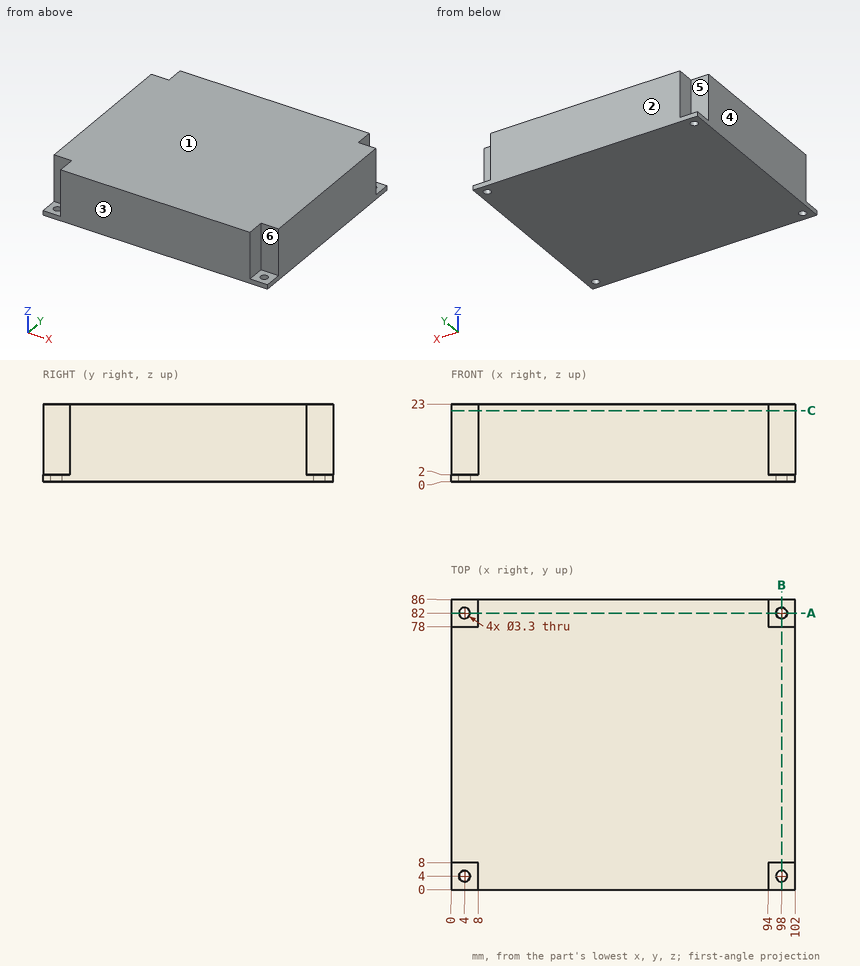
Design review of the part shown in the three views and the two pictorial views. Dimensions are in mm from the part's minimum x, y and z. A direction names the side the tool comes from. Give positions to 0.01 mm unless a question says otherwise; leave off trailing zeros. Write each loop counter-clockwise with the first axis right and the second up, starting at its lowest first coordinate (ties: lowest second). Pieces come first, ordered by that corner, then holes. Notation, with made-up numbers: M 17.5,43 L 25.5,43 A13 cw 25.5,64 Z; hole C -11.5,53 d6. An arc over 180 degrees is marked long. Return JSON: item names as keys, results as strings. Group by question number.
Item 1: Wall thickness on line 1 along Y through (x, z) = (4, 1.2); line 2 along X through (y, z) = (4, 0.85); line 3 along X through (y, z) = (81.5, 6.75): over which ranges is each line inside the solid? List them lowest first.
Item 2: Take a section at B-B (x = 98). Give the boundary of the cut face in (y, z), plus the area to 3 significant figures.
Item 3: Clearance check with flat-ended pins moving along their axes: pin 1 Ø2.5 at (x, y) = (3, 3) entering from +Z; pin 2 Ø6.5 at (x, z) = (98.5, 7.5) entering from -Y; pin 3 Ø4 at (x, z) = (5, 12.5) entering from +Y. State where each tip first meets the part, or that it passes through.
Item 4: The part is to be moulded in two halves that separate along Y. For the marked faces 1, 2 and 3, say which applies: pulls with the +Y half, pulls with the -Y half, needs draft (parallel to the pull), parting line crosses it, or undercut.
Item 5: Tool access review of the marked faces 4, 5 and 6: name each direction out of +Z, -Z, +X, -X, +Y, -Y from which nothing blocks a thin tool from reaching the whole face with its end or side.
Item 6: Take a section at A-A (y = 82). Give the boundary of the cut face in (x, z).
Item 7: Take a section at C-C (z = 21). Give the boundary of the cut face in (x, y).
Return value:
{
 "1": {"line 1": "y = 0 to 2.35, 5.65 to 80.35, 83.65 to 86", "line 2": "x = 0 to 2.35, 5.65 to 96.35, 99.65 to 102", "line 3": "x = 8 to 94"},
 "2": {"outline": "M 0,0 L 2.35,0 L 2.35,2 L 0,2 Z; M 5.65,0 L 80.35,0 L 80.35,2 L 78,2 L 78,23 L 8,23 L 8,2 L 5.65,2 Z; M 83.65,0 L 86,0 L 86,2 L 83.65,2 Z", "area": "1,630 mm2"},
 "3": {"pin 1": "stops at z = 2", "pin 2": "stops at y = 8", "pin 3": "stops at y = 78"},
 "4": {"face 1": "needs draft", "face 2": "pulls with the +Y half", "face 3": "pulls with the -Y half"},
 "5": {"face 4": "+Z, -Z, -X, +Y, -Y", "face 5": "+Z, -X, +Y", "face 6": "+Z, +X, -Y"},
 "6": {"outline": "M 0,0 L 2.35,0 L 2.35,2 L 0,2 Z; M 5.65,0 L 96.35,0 L 96.35,2 L 94,2 L 94,23 L 8,23 L 8,2 L 5.65,2 Z; M 99.65,0 L 102,0 L 102,2 L 99.65,2 Z"},
 "7": {"outline": "M 0,8 L 8,8 L 8,0 L 94,0 L 94,8 L 102,8 L 102,78 L 94,78 L 94,86 L 8,86 L 8,78 L 0,78 Z"}
}
